Part print with two shaded views. Sizes in mm from the minimum x, y, z corner. A direction names the side the tool comes from. Coordinates: 2 decimals unless noted, no trailing zeros. Loops run counter-clockwise (first coordinate to the right, second up) from the corner with the lowest first, then second, coordinate; pieces in that order, holes last.
(1) Wall check: L1, parallel to Y at x = 22, z = 11; L2, parallel to X at y = 23, z = 43; L3, parallel to Y at x = 22.5, z = 82.5. Give the ranges that are in metal, low to high.
(2) Slice it at A-A (x = 22.5). Give the cut face in (y, z).
(3) Tool access for the marked faces 5 and 6: list every direction of +Z, -Z, +X, -X, +Y, -Y with a clear straight run to the whole face (end or side of a thin tool).
(4) Flat gauge pins, fed straight in: P1, Ø2, axis at x = 13, y = 82, coming from the -Z side; P2, Ø10, axis at y = 77.5, z = 8.5, coming from the -X side; P3, Ø12, axis at x = 34.5, y = 83.5, coming from the +Z side; P4, Ø10, axis at x = 17.5, z = 35, coming from the -Y side. Where does each tip first touch, or does it go through?
(5) Slice it at C-C (y = 22.5). Give the cut face in (x, z), and give its area (3 significant figures).
(6) Slice it at D-D (x = 10). Give the cut face in (y, z).
(7) Two-plate mould, pull along X, no slides. Class the marked faces 1, 2, 3 and 4: pulls with the +X half, pulls with the -X half, needs draft (parallel to the pull), parting line crosses it, or undercut.
(8) Slice it at B-B (y = 122.5). Give the cut face in (x, z), and give its area (3 significant figures).
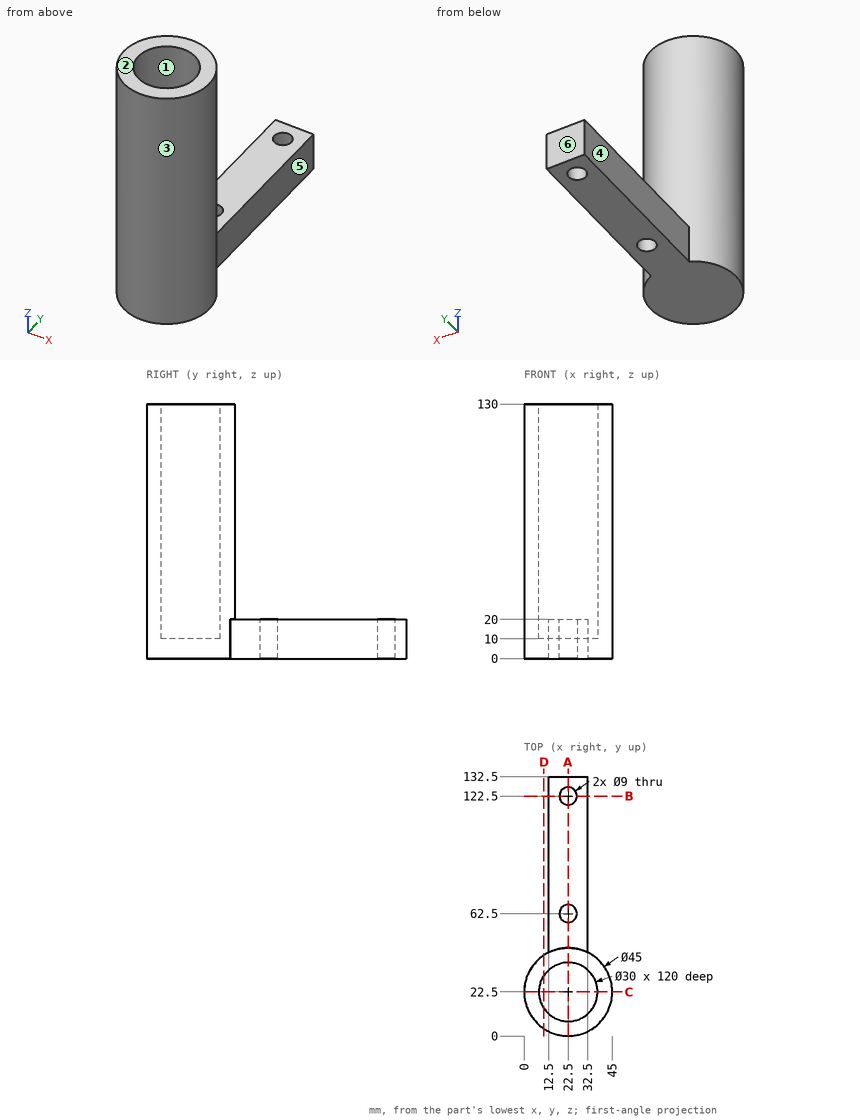
Response values:
1. L1: y = 0.01 to 7.51, 37.49 to 58.03, 66.97 to 118.03, 126.97 to 132.5
1. L2: x = 0.01 to 7.51, 37.49 to 44.99
1. L3: y = 0 to 7.5, 37.5 to 45
2. outline: (0, 0) - (58, 0) - (58, 20) - (45, 20) - (45, 130) - (37.5, 130) - (37.5, 10) - (7.5, 10) - (7.5, 130) - (0, 130) - close; (67, 0) - (118, 0) - (118, 20) - (67, 20) - close; (127, 0) - (132.5, 0) - (132.5, 20) - (127, 20) - close
3. face 5: +Z, -Z, +X, +Y
3. face 6: +Z, -Z, +X, -X, +Y
4. P1: stops at z = 0
4. P2: stops at x = 12.5
4. P3: stops at z = 20
4. P4: stops at y = 0
5. outline: (0, 0) - (45, 0) - (45, 130) - (37.5, 130) - (37.5, 10) - (7.5, 10) - (7.5, 130) - (0, 130) - close
5. area: 2,250 mm2
6. outline: (3.79, 0) - (41.21, 0) - (41.21, 130) - (30.79, 130) - (30.79, 10) - (14.21, 10) - (14.21, 130) - (3.79, 130) - close
7. face 1: undercut
7. face 2: needs draft
7. face 3: parting line crosses it
7. face 4: pulls with the -X half
8. outline: (12.5, 0) - (18, 0) - (18, 20) - (12.5, 20) - close; (27, 0) - (32.5, 0) - (32.5, 20) - (27, 20) - close
8. area: 220 mm2
